```python
from build123d import *

# Parameters (mm, degrees)
F0_W     = 80
F0_H     = 6
F0_R     = 1.25
F1_DEPTH = 9
F0_H_2   = 2.5
F2_DEPTH = 5
F4_DEPTH = 80
F5_SIZE  = 0.5
F6_SIZE  = 1


with BuildPart() as f1:
    # F0 (on Top) → F1 (new body)
    with BuildSketch(Plane.XY):
        Rectangle(F0_W, F0_H)
        with Locations((-20, 0)):
            Circle(F0_R, mode=Mode.SUBTRACT)
        with Locations((20, 0)):
            Circle(F0_R, mode=Mode.SUBTRACT)
    extrude(amount=F1_DEPTH)

    # F0 (on Top) → F2 (join)
    with BuildSketch(Plane.XY):
        with Locations((0, -4.25)):
            Rectangle(F0_W, F0_H_2)
        with Locations((0, 4.25)):
            Rectangle(F0_W, F0_H_2)
    extrude(amount=F2_DEPTH)

    # F3 (on face) → F4 (cut)
    with BuildSketch(Plane.YZ.offset(40)):
        with BuildLine():
            Line((-4, 0), (4, 0))
            ThreePointArc((4, 0), (0, 2.5), (-4, 0))
        make_face()
    extrude(amount=-F4_DEPTH, mode=Mode.SUBTRACT)

    # F5
    f5_edges = [f1.edges().sort_by_distance(p)[0] for p in [
        (-21.25, 0, 9),
        (18.75, 0, 9),
    ]]
    chamfer(f5_edges, length=F5_SIZE)

    # F6
    f6_edges = [f1.edges().sort_by_distance(p)[0] for p in [
        (40, 4.25, 5),
        (40, 5.5, 2.5),
        (40, 3, 7),
        (40, 0, 9),
        (40, -3, 7),
        (40, -4.25, 5),
        (40, -5.5, 2.5),
    ]]
    chamfer(f6_edges, length=F6_SIZE)


solid = f1.part
```
Geometry: final body of the model. Coordinates: model frame, mm. A direction names the side the tool comes from. Round coordinates to 2 decimals unless told otherwise and drop trailing zeros. Order: outer loops, then holes, each group sorted by start corner. A loop starts at its lowest first (then second) coordinate and runs counter-clockwise, first axis right, second up. Notation, with made-up numbers: (-26, 87.25) -> (3, 87.25) arc R22 cw to (3, 94.25) -> close; hole circle Ø10 at (28, -31.75). An arc over 180 degrees is marked (long way). Use one line per item in the form item = value.
(1) Section B-B on z = 7.25. Return loops of the section in (x, y).
Results list:
outline = (-40, -3) -> (39, -3) -> (40, -2) -> (40, 2) -> (39, 3) -> (-40, 3) -> close; hole circle Ø2.5 at (-20, 0); hole circle Ø2.5 at (20, 0)
(2) Access query for faces 1 (the face through (-1, -4, 5)), 2 (the face through (-1, 4, 5)), 3 (the face through (0.6, 0.1, 2.5)). Directions: +Z, -Z, +X, -X, +Y, -Y. A direction counts if a zero-diameter tool reaches every point of the face in a straight line with its end or side. Return the directions, or none.
Results list:
face_1 = +Z, +X, -X, -Y
face_2 = +Z, +X, -X, +Y
face_3 = -Z, +X, -X
(3) Section D-D on z = 1.5. Return loops of the section in (x, y), and give its area (3 significant figures).
Results list:
outline = (-40, -5.5) -> (39, -5.5) -> (40, -4.5) -> (40, -2.81) -> (-40, -2.81) -> close; (-40, 2.81) -> (40, 2.81) -> (40, 4.5) -> (39, 5.5) -> (-40, 5.5) -> close
area = 429 mm^2
(4) Section A-A on x = -20. Return loops of the section in (y, z), and give its area (3 significant figures).
Results list:
outline = (-5.5, 0) -> (-4, 0) arc R4.45 cw to (-1.25, 2.32) -> (-1.25, 8.5) -> (-1.75, 9) -> (-3, 9) -> (-3, 5) -> (-5.5, 5) -> close; (1.25, 2.32) arc R4.45 cw to (4, 0) -> (5.5, 0) -> (5.5, 5) -> (3, 5) -> (3, 9) -> (1.75, 9) -> (1.25, 8.5) -> close
area = 48.0 mm^2
(5) Ray query, probe 1 along X at (y, z) = (0, 6); probe 2 along X at (y, z) = (-1, 8.5); probe 3 along Y at (x, z) = (-20, 7). Return the intervals inside material, ascending. Write a range as [from, to].
Results list:
probe_1 = [-40, -21.25], [-18.75, 18.75], [21.25, 40]
probe_2 = [-40, -20.75], [-19.25, 19.25], [20.75, 39.5]
probe_3 = [-3, -1.25], [1.25, 3]
(6) Draft query along Y for faces 4 (the face through (-1, -3, 7)), 5 (the face through (-18.845, -0.479, 5.367)), 6 (the face through (-1, 3, 7)), 7 (the face through (-1, 5, 0)). Return one class per face: pulls with the +Y half, pulls with the -Y half, needs draft (parallel to the pull), parting line crosses it, or undercut.
Results list:
face_4 = pulls with the -Y half
face_5 = undercut
face_6 = pulls with the +Y half
face_7 = needs draft
(7) Section C-C on y = 0. Return loops of the section in (x, z).
Results list:
outline = (-40, 2.5) -> (-21.25, 2.5) -> (-21.25, 8.5) -> (-21.75, 9) -> (-40, 9) -> close; (-18.75, 2.5) -> (18.75, 2.5) -> (18.75, 8.5) -> (18.25, 9) -> (-18.25, 9) -> (-18.75, 8.5) -> close; (21.25, 2.5) -> (40, 2.5) -> (40, 8) -> (39, 9) -> (21.75, 9) -> (21.25, 8.5) -> close
(8) First-contact query: pin 1 Ø2 at (x, y) = (-11, 2.5) entering from -Z; pin 2 Ø1.5 at (x, y) = (-20, 0) entering from +Z; pin 3 Ø2 at (x, z) = (8.5, 8) entering from -Y; pin 4 Ø1.2 at (x, z) = (12, 8) entering from +Y. Flat tips, straight axial feed; report the tip coordinate or a pass-through.
Results list:
pin_1 = 0.8
pin_2 = through
pin_3 = -3
pin_4 = 3
